Here's how the part is built. I have some questions about the finished solid (model axes, mm). Give positions to 0.01 mm unless a question says otherwise; leave off trailing zeros. Loops run counter-clockwise (first coordinate to the right, second up) from the corner with the lowest first, then second, coordinate; pieces in that order, holes last. Notation, with made-up numbers: (79, 61.25) -> (92, 61.25) arc R16 cw to (92, 81.25) -> close; hole circle Ø5 at (-14.5, 41.5). An arc over 180 degrees is marked (long way). Answer in a Markdown table with one row per item. Add a question column.
Item 1: If I drill on line 1 (Y direction, x = 12.7, z = -2.3); line 2 (X direction, y = 8.5, z = -12.7) (3 decimals); line 3 (X direction, y = 19.05, z = -2.7), over which ranges is the centre line in solid material (lowest first)?
Item 2: If we section it at D-D (y = 7): Write out the boundary of the cut face in (x, z) (3 decimals).
Item 3: If we section it at C-C (x = 20): Write out the boundary of the cut face in (y, z), then the cut area to 3 significant figures.
Item 4: If we section it at A-A (z = -12.7): Write out the boundary of the cut face in (x, y) (3 decimals).
Item 5: We'd pull the mould along X, two halves only. Please class faces 1 (the face through (10.15, 19.16, -1.74)), 2 (the face through (9.839, 18.783, -21.785)), 3 (the face through (0, 19, -13)), 4 (the face through (18, 38.1, -4)): released by +X, released by -X, zero draft, split by the parting line, or undercut.
Item 6: If we section it at B-B (x = 12.7): Write out the boundary of the cut face in (y, z) (3 decimals).
```python
from build123d import *

# Parameters (mm, degrees)
SKETCH1_W                        = 25.4
SKETCH1_H                        = 25.4
SKETCH1_R                        = 9.525
BOSS_EXTRUDE1_DEPTH              = 38.1
TAP_DRILL_FOR_1_4_20_TAP1_REACH  = 54.363
TAP_DRILL_FOR_1_4_20_TAP1_BORE_R = 2.5527


with BuildPart() as part:
    # Sketch1 → Boss-Extrude1 (new body)
    with BuildSketch(Plane(origin=(0, 0, 0), x_dir=(1, 0, 0), z_dir=(0, 1, 0))):
        with Locations((12.7, 12.7)):
            Rectangle(SKETCH1_W, SKETCH1_H)
        with Locations(Location((12.7, 12.7, 0), (0, 0, 90))):
            Circle(SKETCH1_R, mode=Mode.SUBTRACT)
    extrude(amount=BOSS_EXTRUDE1_DEPTH)

    # Tap Drill for 1/4-20 Tap1 bore → Tap Drill for 1/4-20 Tap1 (cut, up to next)
    with BuildSketch(Plane.XY, mode=Mode.PRIVATE) as tap_drill_for_1_4_20_tap1_sk1:
        with Locations((12.7, 19.05)):
            Circle(TAP_DRILL_FOR_1_4_20_TAP1_BORE_R)
    tap_drill_for_1_4_20_tap1_tool1 = extrude(tap_drill_for_1_4_20_tap1_sk1.sketch, amount=-TAP_DRILL_FOR_1_4_20_TAP1_REACH, mode=Mode.PRIVATE) & part.part
    add(tap_drill_for_1_4_20_tap1_tool1.solids().sort_by_distance((12.7, 19.05, 0))[0], mode=Mode.SUBTRACT)


solid = part.part
```
Recorded:
| question | item | result |
|---|---|---|
| 1 | line 1 | y = 0 to 16.5, 21.6 to 38.1 |
| 1 | line 2 | x = 0 to 3.175, 22.225 to 25.4 |
| 1 | line 3 | x = 0 to 10.15, 15.25 to 25.4 |
| 2 | outline | (0, -25.4) -> (25.4, -25.4) -> (25.4, 0) -> (0, 0) -> close; hole circle Ø19.05 at (12.7, -12.7) |
| 3 | outline | (0, -25.4) -> (38.1, -25.4) -> (38.1, -18.82) -> (0, -18.82) -> close; (0, -6.58) -> (38.1, -6.58) -> (38.1, 0) -> (0, 0) -> close |
| 3 | area | 502 mm^2 |
| 4 | outline | (0, 0) -> (3.175, 0) -> (3.175, 38.1) -> (0, 38.1) -> close; (22.225, 0) -> (25.4, 0) -> (25.4, 38.1) -> (22.225, 38.1) -> close |
| 5 | face 1 | undercut |
| 5 | face 2 | undercut |
| 5 | face 3 | released by -X |
| 5 | face 4 | zero draft |
| 6 | outline | (0, -25.4) -> (38.1, -25.4) -> (38.1, -22.225) -> (0, -22.225) -> close; (0, -3.175) -> (16.497, -3.175) -> (16.497, 0) -> (0, 0) -> close; (21.603, -3.175) -> (38.1, -3.175) -> (38.1, 0) -> (21.603, 0) -> close |
